Geometry: final body of the model. Coordinates: model frame, mm. Face numbers are marked on the shaded views. A direction names the side the tool comes from. Coordinates: 2 decimals unless noted, no trailing zeros. Write each loop counter-clockwise with the first axis right and the second up, starting at its lowest first coordinate (ties: lowest second). Pieces come first, ordered by that corner, then holes. Notation, with made-up numbers: (-36, 43.25) -> (13, 43.25) arc R12 ccw to (13, 54.25) -> close; hole circle Ø3 at (-24, 62.25). An arc over 180 degrees is marked (long way). One line per item, written item: value.
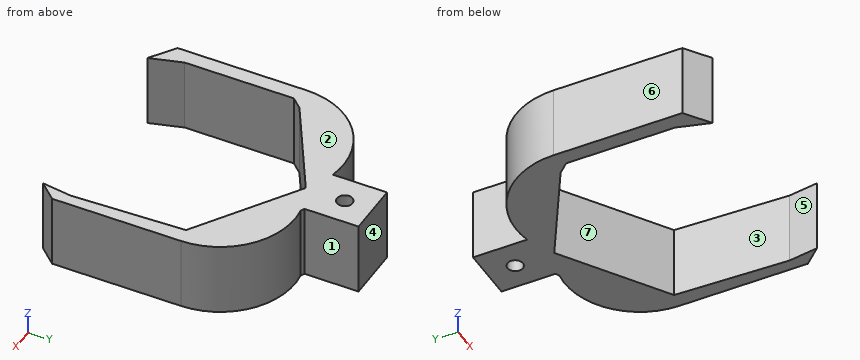
```python
from build123d import *

# Parameters (mm, degrees)
F0_R     = 2.663463
F1_DEPTH = 25.4
F2_DEPTH = 25.4


with BuildPart() as f1:
    # F0 (on Top) → F1 (new body)
    with BuildSketch(Plane.XY):
        with BuildLine():
            ThreePointArc((-9.537551, 54.887395), (-32.102884, 49.673264), (-42.132925, 28.797926))
            Line((-42.132925, 28.797926), (-42.132925, -15.462926))
            Line((-42.132925, -15.462926), (-33.588473, -21.421118))
            Line((-33.588473, -21.421118), (-36.878168, -10.327116))
            Line((-36.878168, -10.327116), (-36.878168, 27.189448))
            Line((-36.878168, 27.189448), (-33.588473, 30.825427))
            Line((-33.588473, 30.825427), (0, 50.559394))
            Line((0, 50.559394), (35.039842, 27.69687))
            Line((35.039842, 27.69687), (36.458459, -11.207074))
            Line((36.458459, -11.207074), (35.039842, -21.421118))
            Line((35.039842, -21.421118), (40.430587, -15.462926))
            Line((40.430587, -15.462926), (40.430587, 28.797926))
            ThreePointArc((40.430587, 28.797926), (31.391675, 48.416927), (10.605718, 54.294944))
            Line((10.605718, 54.294944), (9.183838, 54.887395))
            Line((9.183838, 54.887395), (9.183838, 73.490292))
            Line((9.183838, 73.490292), (-9.537551, 73.490292))
            Line((-9.537551, 73.490292), (-9.537551, 54.887395))
        make_face()
        with Locations((0, 63.979626)):
            Circle(F0_R, mode=Mode.SUBTRACT)
    extrude(amount=F1_DEPTH)

    # F0 (on Top) → F2 (join)
    with BuildSketch(Plane.XY):
        with BuildLine():
            ThreePointArc((-9.537551, 54.887395), (-32.102884, 49.673264), (-42.132925, 28.797926))
            Line((-42.132925, 28.797926), (-42.132925, -15.462926))
            Line((-42.132925, -15.462926), (-33.588473, -21.421118))
            Line((-33.588473, -21.421118), (-36.878168, -10.327116))
            Line((-36.878168, -10.327116), (-36.878168, 27.189448))
            Line((-36.878168, 27.189448), (-33.588473, 30.825427))
            Line((-33.588473, 30.825427), (0, 50.559394))
            Line((0, 50.559394), (35.039842, 27.69687))
            Line((35.039842, 27.69687), (36.458459, -11.207074))
            Line((36.458459, -11.207074), (35.039842, -21.421118))
            Line((35.039842, -21.421118), (40.430587, -15.462926))
            Line((40.430587, -15.462926), (40.430587, 28.797926))
            ThreePointArc((40.430587, 28.797926), (31.391675, 48.416927), (10.605718, 54.294944))
            Line((10.605718, 54.294944), (9.183838, 54.887395))
            Line((9.183838, 54.887395), (9.183838, 73.490292))
            Line((9.183838, 73.490292), (-9.537551, 73.490292))
            Line((-9.537551, 73.490292), (-9.537551, 54.887395))
        make_face()
        with Locations((0, 63.979626)):
            Circle(F0_R, mode=Mode.SUBTRACT)
    extrude(amount=F2_DEPTH)


solid = f1.part
```
(1) Pull-direction query (X, two-part tool) for the marked faces 4, 5, 6 and 7; classes: released by +X, released by -X, zero draft, split by the parting line, or undercut.
Responses:
face 4: zero draft
face 5: undercut
face 6: released by -X
face 7: undercut
(2) Section B-B (z = 6.25). Return the cut outline in (x, y), then the cut area to 3 significant figures.
Responses:
outline: (-42.13, -15.46) -> (-33.59, -21.42) -> (-36.88, -10.33) -> (-36.88, 27.19) -> (-33.59, 30.83) -> (0, 50.56) -> (35.04, 27.7) -> (36.46, -11.21) -> (35.04, -21.42) -> (40.43, -15.46) -> (40.43, 28.8) arc R25.81 ccw to (10.61, 54.29) -> (9.18, 54.89) -> (9.18, 73.49) -> (-9.54, 73.49) -> (-9.54, 54.89) arc R26.74 ccw to (-42.13, 28.8) -> close; hole circle Ø5.33 at (0, 63.98)
area: 1,910 mm2
(3) Section A-A (y = 65.5). Return the cut outline in (x, z), then the cut area to 3 significant figures.
Responses:
outline: (-9.54, 0) -> (-2.19, 0) -> (-2.19, 25.4) -> (-9.54, 25.4) -> close; (2.19, 0) -> (9.18, 0) -> (9.18, 25.4) -> (2.19, 25.4) -> close
area: 364 mm2
(4) Reachability of the marked faces 1, 2 and 3 from +Z, -Z, +X, -X, +Y, -Y: full face, straight path, thin tool, end or side. Return the list, or none.
Responses:
face 1: +Z, -Z, +X, +Y
face 2: +Z, +X, -X, +Y, -Y
face 3: +Z, -Z
(5) Section D-D (x = -17.5). Return the cut outline in (y, z).
Responses:
outline: (40.28, 0) -> (55.45, 0) -> (55.45, 25.4) -> (40.28, 25.4) -> close
(6) First-contact query: pin 1 (6 mm diameter, centred on x = -21, z = 17, fed in from -Y); pin 2 (12 mm diameter, centred on x = -19, z = 10, fed in from -Y); pin 3 (5.5 mm diameter, centred on y = 61.5, z = 6.5, fed in from -X). Flat tips, straight axial feed; report the tip coordinate or a pass-through.
Responses:
pin 1: stops at y = 36.46
pin 2: stops at y = 35.87
pin 3: stops at x = -9.54
(7) Section C-C (y = 4.5). Return the cut outline in (x, z).
Responses:
outline: (-42.13, 0) -> (-36.88, 0) -> (-36.88, 25.4) -> (-42.13, 25.4) -> close; (35.89, 0) -> (40.43, 0) -> (40.43, 25.4) -> (35.89, 25.4) -> close
(8) Line query: line 1 (Y direction, x = 0, z = 12.5); line 2 (X direction, y = 69.5, z = 3.75); line 3 (X direction, y = 34.5, z = 5.25). Output: solid intervals per line, ascending. Write a range as [from, to].
Responses:
line 1: y = [50.56, 61.32], [66.64, 73.49]
line 2: x = [-9.54, 9.18]
line 3: x = [-41.52, -27.33], [24.61, 39.79]
